```python
from build123d import *

# Parameters (mm, degrees)
BOSS_EXTRUDE1_DEPTH = 25.4
BOSS_EXTRUDE2_DEPTH = 2.54
FILLET1_R           = 2.54
SKETCH3_R           = 1.524
BOSS_EXTRUDE3_DEPTH = 2.54
SKETCH4_R           = 1.524
SKETCH4_W           = 3.81
SKETCH4_H           = 8.89
BOSS_EXTRUDE4_DEPTH = 2.54
CUT_EXTRUDE1_REACH  = 37.786
SKETCH5_W           = 6.027706616
SKETCH5_H           = 19.671501998
SKETCH6_W           = 3.81
SKETCH6_H           = 12.7
BOSS_EXTRUDE5_DEPTH = 25.4


with BuildPart() as part:
    # Sketch1 → Boss-Extrude1 (new body)
    with BuildSketch(Plane(origin=(0, 0, 0), x_dir=(1, 0, 0), z_dir=(0, 1, 0))):
        Polygon((-12.7, 6.35), (-5.08, 6.35), (-5.08, 4.445), (-8.89, 4.445), (-8.89, -4.445), (8.89, -4.445), (8.89, 4.445), (5.08, 4.445), (5.08, 6.35), (12.7, 6.35), (12.7, -6.35), (-12.7, -6.35), align=None)
    extrude(amount=BOSS_EXTRUDE1_DEPTH)

    # Sketch2 → Boss-Extrude2 (add)
    with BuildSketch(Plane.XZ):
        Polygon((-12.7, -6.35), (-19.05, -6.35), (-19.05, 22.86), (19.05, 22.86), (19.05, -6.35), (12.7, -6.35), (5.08, -6.35), (5.08, -4.445), (8.89, -4.445), (8.89, 4.445), (-8.89, 4.445), (-8.89, -4.445), (-5.08, -4.445), (-5.08, -6.35), align=None)
    extrude(amount=BOSS_EXTRUDE2_DEPTH)

    # Fillet1
    fillet1_edges = [part.edges().sort_by_distance(p)[0] for p in [
        (12.7, 0, 0),
        (0, 0, 6.35),
        (-12.7, 0, 0),
    ]]
    fillet(fillet1_edges, radius=FILLET1_R)

    # Sketch3 → Boss-Extrude3 (add)
    with BuildSketch(Plane.XZ.offset(2.54)):
        with Locations(Location((-13.8176, -0.4318, 0), (0, 0, 270))):
            Circle(SKETCH3_R)
    boss_extrude3 = extrude(amount=BOSS_EXTRUDE3_DEPTH)

    # Sketch4 → Boss-Extrude4 (add)
    with BuildSketch(Plane(origin=(0, -2.54, 0), x_dir=(-1, 0, 0), z_dir=(0, -1, 0))):
        with Locations(Location((13.8176, -20.1168, 0), (0, 0, 90))):
            Circle(SKETCH4_R)
        with Locations((13.8176, -10.541)):
            Rectangle(SKETCH4_W, SKETCH4_H)
    boss_extrude4 = extrude(amount=BOSS_EXTRUDE4_DEPTH)

    # Mirror1: Boss-Extrude3, Boss-Extrude4 across plane
    add(boss_extrude3.mirror(Plane(origin=(0, 0, 0), x_dir=(0, 0, 1), z_dir=(1, 0, 0))))
    add(boss_extrude4.mirror(Plane(origin=(0, 0, 0), x_dir=(0, 0, 1), z_dir=(1, 0, 0))))

    # Sketch5 → Cut-Extrude1 (cut, up to next)
    with BuildSketch(Plane.XY.offset(6.35), mode=Mode.PRIVATE) as cut_extrude1_sk1:
        with Locations((4.765146447, 12.644392592)):
            Rectangle(SKETCH5_W, SKETCH5_H)
    cut_extrude1_tool1 = extrude(cut_extrude1_sk1.sketch, amount=-CUT_EXTRUDE1_REACH, mode=Mode.PRIVATE) & part.part
    add(cut_extrude1_tool1.solids().sort_by_distance((4.765146, 12.644393, 6.35))[0], mode=Mode.SUBTRACT)

    # Sketch6 → Boss-Extrude5 (add)
    with BuildSketch(Plane(origin=(0, 25.4, 0), x_dir=(1, 0, 0), z_dir=(0, 1, 0))):
        with Locations((-10.795, 0)):
            Rectangle(SKETCH6_W, SKETCH6_H)
        with Locations((10.795, 0)):
            Rectangle(SKETCH6_W, SKETCH6_H)
    extrude(amount=BOSS_EXTRUDE5_DEPTH)


solid = part.part
```
Part model, mm, in its own coordinate system. A direction names the side the tool comes from. Give positions to 0.01 mm unless a question says otherwise; leave off trailing zeros. Write each loop counter-clockwise with the first axis right and the second up, starting at its lowest first coordinate (ties: lowest second). Pieces come first, ordered by that corner, then holes. Notation, with made-up numbers: (38, 54) -> (74, 54) arc R25 cw to (74, 90) -> close; hole circle Ø4 at (-10, 77). An arc over 180 degrees is marked (long way). Put each result on its own line as item: value. Start each with the question number.
Item 1: Cut at D-D (x = -6). List the corners of the cut face in (y, z) (3 decimals), then the cut area to 3 significant figures.
Item 2: Cut at B-B (y = 43). List the corners of the cut face in (x, z), then the cut area to 3 significant figures.
Item 3: Cut at C-C (z = 5.25). List the corners of the cut face in (x, y), then the cut area to 3 significant figures.
Item 4: Wall check: L1, parallel to X at y = 17, z = -4.5; L2, parallel to X at y = 29, z = 5; L3, parallel to Y at x = 4, z = 17.5. Give the ranges that are in metal, low to high. Write a range as [from, to].
Item 5: Pull direction Z, two halves, no side cores. Call faces 1 (the face through (0, -1, 22.86)), 2 (the face through (-15.305, -3.792, -0.101)), 3 (the face through (5, 2.809, 5)): pulls with the +Z half, pulls with the -Z half, needs draft (parallel to the pull), parting line crosses it, or undercut.
Item 6: Pin check, flat tips, straight feed: pin 1 Ø2 at (x, z) = (13, 13) entering from +Y; pin 2 Ø1 at (x, z) = (5, 6) entering from -Y; pin 3 Ø3 at (y, z) = (-4.5, 12.5) entering from -X. Stop position of each tip, or through.
Item 7: Cut at A-A (x = 7). List the corners of the cut face in (y, z) (3 decimals), then the cut area to 3 significant figures.
Item 8: Which spindle directions (+Z, -Z, +X, -X, +Y, -Y) get a long thin tool onto all of the face, cutting with end or side? Do faces 4 (the face through (11.913, -4, 11)), 5 (the face through (-14, -4, 6.096)), 6 (the face through (15.305, -3.792, -0.101)). Say none if no direction does.
Answer list:
1. outline: (-2.54, -6.35) -> (25.4, -6.35) -> (25.4, -4.445) -> (-2.54, -4.445) -> close; (-2.54, 4.445) -> (25.4, 4.445) -> (25.4, 6.35) -> (2.54, 6.35) arc R2.54 cw to (0, 8.89) -> (0, 22.86) -> (-2.54, 22.86) -> close
1. area: 150 mm2
2. outline: (-12.7, -6.35) -> (-8.89, -6.35) -> (-8.89, 6.35) -> (-12.7, 6.35) -> close; (8.89, -6.35) -> (12.7, -6.35) -> (12.7, 6.35) -> (8.89, 6.35) -> close
2. area: 96.8 mm2
3. outline: (-19.05, -2.54) -> (19.05, -2.54) -> (19.05, 0) -> (15.24, 0) arc R2.54 cw to (12.7, 2.54) -> (12.7, 50.8) -> (8.89, 50.8) -> (8.89, 25.4) -> (-8.89, 25.4) -> (-8.89, 50.8) -> (-12.7, 50.8) -> (-12.7, 2.54) arc R2.54 cw to (-15.24, 0) -> (-19.05, 0) -> close; hole (1.75, 2.81) -> (7.78, 2.81) -> (7.78, 22.48) -> (1.75, 22.48) -> close
3. area: 820 mm2
4. L1: x = [-12.7, -5.08], [5.08, 12.7]
4. L2: x = [-12.7, -8.89], [8.89, 12.7]
4. L3: y = [-2.54, 0]
5. face 1: pulls with the +Z half
5. face 2: undercut
5. face 3: needs draft
6. pin 1: stops at y = 0
6. pin 2: stops at y = -2.54
6. pin 3: stops at x = -15.72
7. outline: (-2.54, -6.35) -> (25.4, -6.35) -> (25.4, -4.445) -> (-2.54, -4.445) -> close; (-2.54, 4.445) -> (2.809, 4.445) -> (2.809, 6.35) -> (2.54, 6.35) arc R2.54 cw to (0, 8.89) -> (0, 22.86) -> (-2.54, 22.86) -> close; (22.48, 4.445) -> (25.4, 4.445) -> (25.4, 6.35) -> (22.48, 6.35) -> close
7. area: 112 mm2
8. face 4: +Z, -Z, -Y
8. face 5: +X, -X, -Y
8. face 6: -Y
